Source: CAD feature listing. Evaluate the final solid. Frame: model axes, mm. Face numbers are marked on the shaded views. A direction names the side the tool comes from. Give positions to 0.01 mm unless a question says otherwise; leave off trailing zeros. Loops run counter-clockwise (first coordinate to the right, second up) from the corner with the lowest first, then second, coordinate; pieces in that order, holes last. Notation, with made-up numbers: M -3.5,-17 L 49.5,-17 A20 cw 49.5,-5 Z; hole C -30,85 d11. An arc over 180 degrees is marked long. Put each result on its own line as item: value. Start each with the question number.
```python
from build123d import *

# Parameters (mm, degrees)
BOSS_EXTRUDE1_START      = -1.2
SKETCH1_R                = 2
BOSS_EXTRUDE1_DEPTH      = 1.3
BOSS_EXTRUDE2_START      = 1
BOSS_EXTRUDE2_DEPTH      = 1.6
BOSS_EXTRUDE3_DEPTH      = 0.9
SKETCH6_R                = 1.5
CUT_EXTRUDE13_DEPTH      = 2.5
BOSS_EXTRUDE4_DEPTH      = 0.0001
BOSS_EXTRUDE4_DEPTH_BACK = 2
SKETCH9_R                = 0.5


with BuildPart() as part:
    # Sketch1 → Boss-Extrude1 (new body)
    with BuildSketch(Plane.XY.offset(BOSS_EXTRUDE1_START)):
        Circle(SKETCH1_R)
    boss_extrude1 = extrude(amount=BOSS_EXTRUDE1_DEPTH)

    # Sketch2 → Boss-Extrude2 (add)
    with BuildSketch(Plane(origin=(0, 0, -1.2), x_dir=(-1, 0, 0), z_dir=(0, 0, -1)).offset(BOSS_EXTRUDE2_START)):
        with BuildLine():
            ThreePointArc((-1.301905334, 1.518236642), (-1.999965901, 0.011678742), (-1.31954734, -1.502928747))
            add(Edge.make_bspline(
                [(-1.301905334, 1.518236642), (-6.689282212, 0.003550345), (-1.31954734, -1.502928747)],
                knots=[0, 0, 0, 1, 1, 1], degree=2))
        make_face()
    boss_extrude2 = extrude(amount=-BOSS_EXTRUDE2_DEPTH)

    # Sketch3 → Boss-Extrude3 (add)
    with BuildSketch(Plane(origin=(0, 0, -2.2), x_dir=(-1, 0, 0), z_dir=(0, 0, -1))):
        with BuildLine():
            Line((-5.337512996, -2.068499627), (-3.337513, -0.746121009))
            add(Edge.make_bspline(
                [(-3.337512996, 0.753381422), (-4.662510017, 0.002619292), (-3.337513, -0.746121009)],
                knots=[0.252652683, 0.252652683, 0.252652683, 0.748987348, 0.748987348, 0.748987348], degree=2))
            Line((-3.337513, 0.753381429), (-13.337512996, 1.031500373))
            Line((-13.337512996, 1.031500373), (-13.337512996, -2.068499627))
            Line((-13.337512996, -2.068499627), (-5.337512996, -2.068499627))
        make_face()
    boss_extrude3 = extrude(amount=-BOSS_EXTRUDE3_DEPTH)

    # Sketch6 → Cut-Extrude13 (cut, symmetric)
    with BuildSketch(Plane.XY.offset(-1.3)):
        with Locations((11.827512996, -0.521079469)):
            Circle(SKETCH6_R)
    cut_extrude13 = extrude(amount=CUT_EXTRUDE13_DEPTH, both=True, mode=Mode.SUBTRACT)

    # Mirror2: Boss-Extrude2, Boss-Extrude3 across plane
    add(boss_extrude2.mirror(Plane(origin=(0, 0, -2.2), x_dir=(1, 0, 0), z_dir=(0, 0, -1))))
    add(boss_extrude3.mirror(Plane(origin=(0, 0, -2.2), x_dir=(1, 0, 0), z_dir=(0, 0, -1))))

    # Mirror3: Boss-Extrude1 across plane
    add(boss_extrude1.mirror(Plane(origin=(0, 0, -2.2), x_dir=(1, 0, 0), z_dir=(0, 0, -1))))

    # Mirror4: Cut-Extrude13 across plane
    add(cut_extrude13.mirror(Plane(origin=(0, 0, -2.2), x_dir=(1, 0, 0), z_dir=(0, 0, -1))), mode=Mode.SUBTRACT)

    # Sketch9 → Boss-Extrude4 (add, two sides: drawn at the far end of the back side and taken through both)
    with BuildSketch(Plane(origin=(0, 0, -3.2), x_dir=(-1, 0, 0), z_dir=(0, 0, -1)).offset(-BOSS_EXTRUDE4_DEPTH_BACK)):
        with BuildLine():
            Line((-11.107531907, -2.068499627), (-7.907531907, -2.068499627))
            Line((-7.907531907, -2.068499627), (-7.907531907, -2.818499627))
            ThreePointArc((-7.907531907, -2.818499627), (-7.995399873, -3.030631662), (-8.207531907, -3.118499627))
            Line((-8.207531907, -3.118499627), (-10.807531907, -3.118499627))
            ThreePointArc((-10.807531907, -3.118499627), (-11.019663942, -3.030631662), (-11.107531907, -2.818499627))
            Line((-11.107531907, -2.818499627), (-11.107531907, -2.068499627))
        make_face()
        with Locations((-10.560929332, -2.601747045)):
            Circle(SKETCH9_R, mode=Mode.SUBTRACT)
        with Locations((-9.510929332, -2.601747045)):
            Circle(SKETCH9_R, mode=Mode.SUBTRACT)
        with Locations((-8.460929332, -2.601747045)):
            Circle(SKETCH9_R, mode=Mode.SUBTRACT)
    extrude(amount=BOSS_EXTRUDE4_DEPTH + BOSS_EXTRUDE4_DEPTH_BACK)


solid = part.part
```
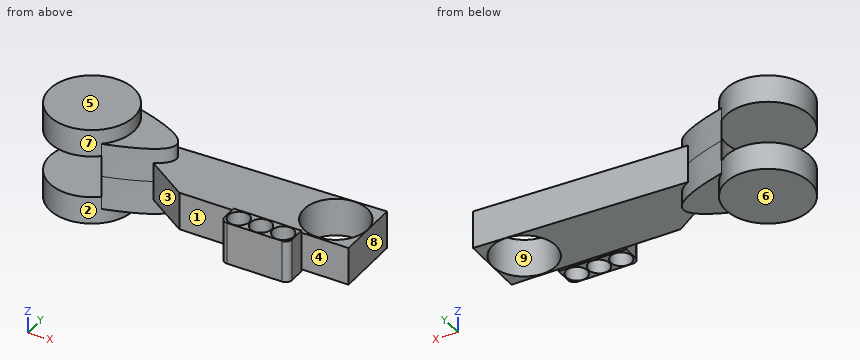
1. Pull-direction query (X, two-part tool) for the marked faces 6, 7, 8 and 9; classes: released by +X, released by -X, zero draft, split by the parting line, or undercut.
2. Set-up query: the marked faces 1, 2, 3, 4 and 5. Return all of +Z, -Z, +X, -X, +Y, -Y with unobstructed straight access to the full face (end or side cutting, diameter ignored); none if empty.
3. Section C-C, the plane x = 7. Output: boundary loops of the cut face in (y, z), plus the area to 3 significant figures.
4. Section B-B, the plane z = -2.4. State how many separate pieces and enclosed holes the cut face has, plus the area to 3 significant figures.
5. Ray query, line 1 (Z direction, x = 1.25, y = -1.35); line 2 (Z direction, x = 2, y = -1.25); line 3 (Z direction, x = 8.25, y = -0.9). Return the intervals inside material, ascending.
6. Contact query for flat-ended pins moving along their axis: pin 1 (3 mm diameter, centred on x = 5, y = 0, fed in from +Z); pin 2 (0.8 mm diameter, centred on y = -2.5, z = -2, fed in from -X); pin 3 (0.8 mm diameter, centred on y = -2.5, z = -2.5, fed in from +X); pin 4 (3 mm diameter, centred on x = 2.5, y = -0.5, fed in from -Z). Output: stop coordinate, or through.
7. Section A-A, the plane x = 0. Output: boundary loops of the cut face in (y, z), plus the area to 3 significant figures.
Results found:
1. face 6: zero draft
1. face 7: split by the parting line
1. face 8: released by +X
1. face 9: undercut
2. face 1: +Z, -Z, -X, -Y
2. face 2: -Z
2. face 3: +Z, -Z, -Y
2. face 4: +Z, -Z, +X, -Y
2. face 5: +Z, +X, -X, +Y, -Y
3. outline: M -2.07,-3.1 L 0.86,-3.1 L 0.86,-1.3 L -2.07,-1.3 Z
3. area: 5.26 mm²
4. separate pieces: 1
4. enclosed holes: 4
4. area: 25.5 mm²
5. line 1: -4.5 to -3.2, -1.2 to 0.1
5. line 2: -3.8 to -0.6
5. line 3: -3.1 to -1.3
6. pin 1: z = -0.6
6. pin 2: x = 7.91
6. pin 3: x = 11.11
6. pin 4: z = -4.5
7. outline: M -2,-4.5 L 2,-4.5 L 2,-3.2 L -2,-3.2 Z; M -2,-1.2 L 2,-1.2 L 2,0.1 L -2,0.1 Z
7. area: 10.4 mm²
